```python
from build123d import *
from OCP.BRepFilletAPI import BRepFilletAPI_MakeChamfer

# Parameters (mm, degrees)
SKETCH1_W           = 20
SKETCH1_H           = 40.56076
BOSS_EXTRUDE1_DEPTH = 9
SKETCH6_R           = 1.35
CUT_EXTRUDE1_DEPTH  = 10
CUT_EXTRUDE2_DEPTH  = 2.5
FILLET1_R           = 2
SKETCH9_R           = 0.8
CUT_EXTRUDE3_DEPTH  = 6.5
SKETCH10_W          = 9
SKETCH10_H          = 7
CUT_EXTRUDE4_DEPTH  = 3.5
CHAMFER1_SIZE       = 2.020725942
CHAMFER1_SIZE_2     = 3.5
FILLET2_R           = 3


# Some blends are built 0.0001 mm under size
with BuildPart() as part:
    # Sketch1 → Boss-Extrude1 (new body)
    with BuildSketch(Plane.XY):
        Rectangle(SKETCH1_W, SKETCH1_H)
    extrude(amount=-BOSS_EXTRUDE1_DEPTH)

    # Sketch6 → Cut-Extrude1 (cut)
    with BuildSketch(Plane(origin=(10, 0, 0), x_dir=(0, 0, -1), z_dir=(1, 0, 0))):
        with Locations(Location((4.3, -15.26519, 0), (0, 0, 180))):
            Circle(SKETCH6_R)
        with Locations((4.3, -5.26519)):
            Circle(SKETCH6_R)
        with Locations((4.3, 15.26519)):
            Circle(SKETCH6_R)
        with Locations(Location((4.3, 5.26519, 0), (0, 0, 180))):
            Circle(SKETCH6_R)
    extrude(amount=-CUT_EXTRUDE1_DEPTH, mode=Mode.SUBTRACT)

    # Sketch8 → Cut-Extrude2 (cut)
    with BuildSketch(Plane.XY):
        with BuildLine():
            Line((-4.488964362, -4.203771991), (-2.672717394, -16.882859941))
            ThreePointArc((-2.672717394, -16.882859941), (0, -19.2), (2.672717394, -16.882859941))
            Line((2.672717394, -16.882859941), (4.488964362, -4.203771991))
            ThreePointArc((4.488964362, -4.203771991), (6.15, 0), (4.488964362, 4.203771991))
            Line((4.488964362, 4.203771991), (2.672717394, 16.882859941))
            ThreePointArc((2.672717394, 16.882859941), (0, 19.2), (-2.672717394, 16.882859941))
            Line((-2.672717394, 16.882859941), (-4.488964362, 4.203771991))
            ThreePointArc((-4.488964362, 4.203771991), (-6.15, 0), (-4.488964362, -4.203771991))
        make_face()
    extrude(amount=-CUT_EXTRUDE2_DEPTH, mode=Mode.SUBTRACT)

    # Fillet1
    # the kernel refuses this fillet: 2 mm, written as the material it takes off along each edge
    with BuildSketch(Plane(origin=(-15, -20.28038, 0), x_dir=(0, 0, -1), z_dir=(1, 0, 0)), Plane(origin=(15, 20.28038, 0), x_dir=(0, 0, -1), z_dir=(-1, 0, 0))) as fillet1_piece_1:
        with BuildLine():
            CenterArc((FILLET1_R, FILLET1_R), FILLET1_R, 180, 90)
            Line((0, FILLET1_R), (0, 0))
            Line((0, 0), (FILLET1_R, 0))
        make_face()
    extrude(amount=30, mode=Mode.SUBTRACT)

    # Sketch9 → Cut-Extrude3 (cut)
    with BuildSketch(Plane.XY.offset(-2.5)):
        with Locations((0, 10)):
            Circle(SKETCH9_R)
        with Locations((0, -10)):
            Circle(SKETCH9_R)
    extrude(amount=-CUT_EXTRUDE3_DEPTH, mode=Mode.SUBTRACT)

    # Sketch10 → Cut-Extrude4 (cut)
    with BuildSketch(Plane.ZY.offset(10)):
        with Locations((-4.5, -10.26517)):
            Rectangle(SKETCH10_W, SKETCH10_H)
    extrude(amount=-CUT_EXTRUDE4_DEPTH, mode=Mode.SUBTRACT)

    # Chamfer1
    chamfer1_edges_1 = [part.edges().sort_by_distance(p)[0] for p in [
        (-10, -6.76517, -4.5),
    ]]
    chamfer1_side_1 = [part.faces().sort_by_distance(p)[0] for p in [
        (-10, -6.724755481, -4.5),
    ]]
    chamfer1_edges_2 = [part.edges().sort_by_distance(p)[0] for p in [
        (-10, -13.76517, -4.5),
    ]]
    chamfer1_side_2 = [part.faces().sort_by_distance(p)[0] for p in [
        (-10, -13.805584519, -4.5),
    ]]
    chamfer1 = BRepFilletAPI_MakeChamfer(part.part.solid().wrapped)
    for e in chamfer1_edges_1:
        chamfer1.Add(CHAMFER1_SIZE - 0.0001, CHAMFER1_SIZE_2 - 0.0001, e.wrapped, chamfer1_side_1[0].wrapped)
    for e in chamfer1_edges_2:
        chamfer1.Add(CHAMFER1_SIZE - 0.0001, CHAMFER1_SIZE_2 - 0.0001, e.wrapped, chamfer1_side_2[0].wrapped)
    add(Compound.cast(chamfer1.Shape()), mode=Mode.REPLACE)  # a hair under: the kernel refuses the full size

    # Fillet2
    fillet2_edges = [part.edges().sort_by_distance(p)[0] for p in [
        (-10, -4.744544058, -4.5),
        (-10, -15.785795942, -4.5),
    ]]
    fillet(fillet2_edges, radius=FILLET2_R)


solid = part.part
```
The listing builds one solid part. Answer for the finished solid, in the listing's coordinates (mm). A direction names the side the tool comes from. Give positions to 0.01 mm unless a question says otherwise; leave off trailing zeros. Loops run counter-clockwise (first coordinate to the right, second up) from the corner with the lowest first, then second, coordinate; pieces in that order, holes last. Notation, with made-up numbers: (31, -24.5) - (61, -24.5) arc R29 cw to (61, 11.5) - close; hole circle Ø7 at (-38, 63). An arc over 180 degrees is marked (long way). Answer as CSV lines item,"result". Start each with the question number.
Item 1: A cutting plane is placed at C-C on x = 5.25. Determine the outline of the cut face in (y, z), then the cut area to 3 significant figures.
Item 2: Find the intervals of material crossed by line 1 (Y direction, x = 2.5, z = -4.3); line 2 (Y direction, x = 5.5, z = -3.25); line 3 (Z direction, x = 6, y = -16.5), in increasing order. Write a range as from..to.
Item 3: A cutting plane is placed at B-B on z = -8. Count the separate pieces of the cut face and the enclosed holes in it, then the cut area to 3 significant figures.
Item 4: Each of these flat-tipped pins is pushed along its axis until it touches: pin 1 (3.5 mm diameter, centred on y = -15.27, z = -4.3, fed in from -X); pin 2 (2 mm diameter, centred on y = -9, z = -4, fed in from -X); pin 3 (2.5 mm diameter, centred on y = -5.27, z = -4.3, fed in from +X). Where does it stop, or does it pass through?
Item 5: For faces 5 (the face through (-3.57, 10.63, -1.23)), 6 (the face through (5.07, -5.21, -2.95)), 7 (the face through (-9.61, -16.04, -4.44)), determine the directions among +Z, -Z, +X, -X, +Y, -Y from which every point of the face is accessible in a straight line to the end or side of a thin tool.
Item 6: The mould has two halves that part along Y. Classify faces 1 (the face through (0, -20.28, -5)), 2 (the face through (5.07, 13.947, -4.007)), 3 (the face through (0, 0, -2.5)), 4 (the face through (-10, -19, -4)): +Y half, -Y half, draft (parallel to the pull), parting line (faces both ways), or undercut.
Item 7: A cutting plane is placed at A-A on y = -10. Determine the outline of the cut face in (x, z).
Found:
1,outline,"(-20.28, -9) - (20.28, -9) - (20.28, -2) arc R2 ccw to (18.28, 0) - (3.2, 0) - (3.2, -2.5) - (-3.2, -2.5) - (-3.2, 0) - (-18.28, 0) arc R2 ccw to (-20.28, -2) - close; hole circle Ø2.7 at (-15.27, -4.3); hole circle Ø2.7 at (-5.27, -4.3); hole circle Ø2.7 at (5.27, -4.3); hole circle Ø2.7 at (15.27, -4.3)"
1,area,"324 mm^2"
2,line 1,"y = -20.28..-16.62, -13.92..-6.62, -3.92..3.92, 6.62..13.92, 16.62..20.28"
2,line 2,"y = -20.28..-16.11, -14.42..-6.11, -4.42..4.42, 6.11..14.42, 16.11..20.28"
2,line 3,"z = -9..-4.85, -3.75..0"
3,separate pieces,"1"
3,enclosed holes,"2"
3,area,"775 mm^2"
4,pin 1,"stops at x = -9.96"
4,pin 2,"stops at x = -6.5"
4,pin 3,"stops at x = 0"
5,face 5,"+Z"
5,face 6,"+X"
5,face 7,"+Z, -Z, -X"
6,face 1,"-Y half"
6,face 2,"undercut"
6,face 3,"undercut"
6,face 4,"draft"
7,outline,"(-6.5, -9) - (-0.8, -9) - (-0.8, -2.5) - (-3.66, -2.5) - (-3.66, 0) - (-6.5, 0) - close; (0.8, -9) - (10, -9) - (10, 0) - (3.66, 0) - (3.66, -2.5) - (0.8, -2.5) - close"
